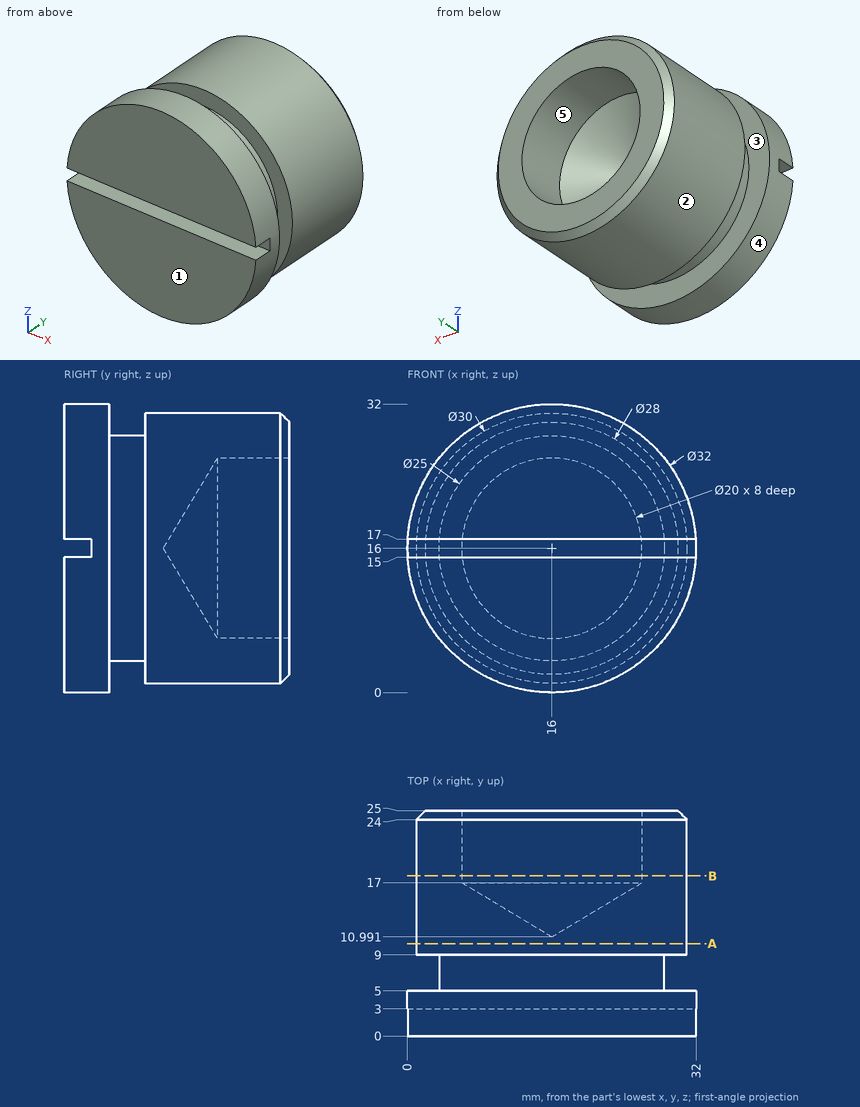
Source: three-view drawing plus pictorial views. Frame: mm from the lowest corner of the part. A direction names the side the tool comes from. Round coordinates to 2 decimals unless told otherwise and drop trailing zeros. Loops run counter-clockwise (first coordinate to the right, second up) from the corner with the lowest first, then second, coordinate; pieces in that order, holes last. Notation, with made-up numbers: M -17,64 L 13,64 A18 ccw 13,88 Z; hole C 56,80.5 d11. An arc over 180 degrees is marked long. Put each result on its own line as item: value. Start each with the question number.
(1) Set-up query: the marked faces 1 and 2. Return all of +Z, -Z, +X, -X, +Y, -Y with unobstructed straight access to the full face (end or side cutting, diameter ignored); none if empty.
(2) Draft query along X for the marked faces 3, 4 and 5. Return one class per face: +X half, -X half, draft (parallel to the pull), parting line (faces both ways), or undercut.
(3) Material intervals for line 1 along X through (y, z) = (21.75, 16); line 2 along Z through (x, y) = (16.5, 1.75), sorted ascending. Write a range as [from, to].
(4) Contact query for flat-ended pins moving along their axis: pin 1 Ø1.5 at (x, z) = (23.5, 12) entering from +Y; pin 2 Ø1 at (x, z) = (18.5, 16) entering from -Y; pin 3 Ø10 at (x, y) = (11.5, 10.5) entering from +Z. Output: stop coordinate, or through.
(5) Section query A-A (y = 10.25). Return loops of the section in (x, z), then the cut area to 3 significant figures.
(6) Section query B-B (y = 17.75). Return loops of the section in (x, z).
Findings below:
1. face 1: +Z, -Z, +X, -X, -Y
1. face 2: +Y
2. face 3: draft
2. face 4: parting line
2. face 5: undercut
3. line 1: x = [1, 6], [26, 31]
3. line 2: z = [0.01, 15], [17, 31.99]
4. pin 1: stops at y = 16.55
4. pin 2: stops at y = 3
4. pin 3: stops at z = 31
5. outline: C 16,16 d30
5. area: 707 mm2
6. outline: C 16,16 d30; hole C 16,16 d20
